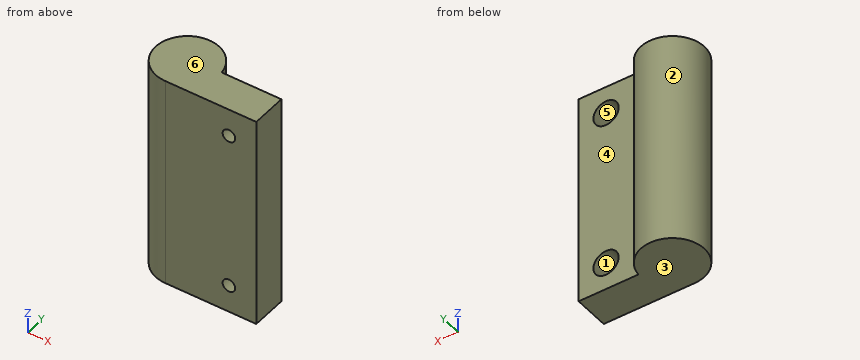
from build123d import *

# Parameters (mm, degrees)
BOSS_EXTRUDE1_DEPTH            = 42.8625
F_8_0_199_DIAMETER_HOLE1_D     = 5.0546
F_8_0_199_DIAMETER_HOLE1_DEPTH = 6.35
F_8_0_199_DIAMETER_HOLE1_TIP   = 1.518555042


with BuildPart() as part:
    # Sketch1 → Boss-Extrude1 (new body)
    with BuildSketch(Plane.XY):
        with BuildLine():
            Line((-19.0864, 25.721816942), (-0.91057904, 25.721816942))
            Line((-0.91057904, 25.721816942), (-0.91057904, 32.833816942))
            Line((-0.91057904, 32.833816942), (-12.854560562, 32.833816942))
            ThreePointArc((-12.854560562, 32.833816942), (-23.919686684, 36.243252538), (-19.0864, 25.721816942))
        make_face()
    extrude(amount=BOSS_EXTRUDE1_DEPTH)

    # #8 (0.199) Diameter Hole1
    with Locations(Plane(origin=(0, 32.833816942, 0), x_dir=(-1, 0, 0), z_dir=(0, 1, 0))):
        with Locations((6.3864, 37.30625), (6.3864, 5.55625)):
            Hole(F_8_0_199_DIAMETER_HOLE1_D / 2, depth=F_8_0_199_DIAMETER_HOLE1_DEPTH)
            with Locations((0, 0, -(F_8_0_199_DIAMETER_HOLE1_DEPTH + F_8_0_199_DIAMETER_HOLE1_TIP / 2))):  # 118° drill point
                Cone(0, F_8_0_199_DIAMETER_HOLE1_D / 2, F_8_0_199_DIAMETER_HOLE1_TIP, mode=Mode.SUBTRACT)


solid = part.part
Here's how the part is built. I have some questions about the finished solid (model axes, mm). Face numbers are marked on the shaded views. A direction names the side the tool comes from. Round coordinates to 2 decimals unless told otherwise and drop trailing zeros. Order: outer loops, then holes, each group sorted by start corner. A loop starts at its lowest first (then second) coordinate and runs counter-clockwise, first axis right, second up. Notation, with made-up numbers: M 1,3 L 7,3 A20 cw 7,9 Z; hole C 71.25,88 d10. An arc over 180 degrees is marked long. One line per question, with ' | ' between items.
1) Imagine slicing it at B-B, the plane z = 26. Write out the boundary of the cut face in (x, y).
Checked values:
outline: M -19.09,25.72 L -0.91,25.72 L -0.91,32.83 L -12.85,32.83 A6.34 ccw long Z
2) I need wall thicknesses on line 1 (Y direction, x = -7.25, z = 18.5); line 2 (X direction, y = 30.25, z = 7); line 3 (X direction, y = 27, z = 38.5). Which ranges of each line are inside material? Lowest first, please.
Checked values:
line 1: y = 25.72 to 32.83 | line 2: x = -25.23 to -8.46, -4.31 to -0.91 | line 3: x = -22.97 to -8.61, -4.16 to -0.91
3) On a 3-axis mill with a long thin cutter (end or side, diameter ignored), from which of +Z, -Z, +X, -X, +Y, -Y can I reach the whole of each face in a straight line? I mean the marked faces 4, 5 and 6. Say none if no direction works.
Checked values:
face 4: +Z, -Z, +X, +Y | face 5: +Y | face 6: +Z, +X, -X, +Y, -Y
4) We'd pull the mould along Z, two halves only. Please class the marked faces 1, 2 and 3: released by +Z, released by -Z, zero draft, split by the parting line, or undercut.
Checked values:
face 1: undercut | face 2: zero draft | face 3: released by -Z
5) Imagine slicing it at A-A, the plane y = 29.5. Write out the boundary of the cut face in (x, z), plus the area to 3 significant figures.
Checked values:
outline: M -24.95,0 L -0.91,0 L -0.91,42.86 L -24.95,42.86 Z; hole C -6.39,5.56 d5.05; hole C -6.39,37.31 d5.05 | area: 990 mm²
6) Imagine slicing it at D-D, the plane y = 31.5. Write out the boundary of the cut face in (x, z).
Checked values:
outline: M -25.47,0 L -0.91,0 L -0.91,42.86 L -25.47,42.86 Z; hole C -6.39,5.56 d5.05; hole C -6.39,37.31 d5.05
7) Imagine slicing it at C-C, the plane x = -6. Count the separate pieces of the cut face and the enclosed holes in it, plus the area to 3 significant figures.
Checked values:
separate pieces: 3 | enclosed holes: 0 | area: 236 mm²
8) I'm going to push flat-ended pins straight in: pin 1 Ø4 at (x, z) = (-6.39, 5.56) entering from +Y; pin 2 Ø9.5 at (x, z) = (-5.5, 14.5) entering from +Y; pin 3 Ø1 at (y, z) = (34, 26) entering from +X. Where does each tip first touch, or does it pass through?
Checked values:
pin 1: stops at y = 26.17 | pin 2: stops at y = 32.83 | pin 3: stops at x = -12.97
